from build123d import *

# Parameters (mm, degrees)
AUFSATZ_LINEAR_AUSTRAGEN1_DEPTH = 15
SKIZZE8_W                       = 15
SKIZZE8_H                       = 1.8
AUFSATZ_LINEAR_AUSTRAGEN2_DEPTH = 3.6
SKIZZE9_W                       = 1.8
SKIZZE9_H                       = 15
AUFSATZ_LINEAR_AUSTRAGEN3_DEPTH = 1.8
SKIZZE10_W                      = 1.8
SKIZZE10_H                      = 15
AUFSATZ_LINEAR_AUSTRAGEN4_DEPTH = 1.8


# Read off the part's stored shape, not the designer's step: Aufsatz-Linear austragen1
with BuildPart() as part:
    # Aufsatz-Linear austragen1 outline → Aufsatz-Linear austragen1 (new body)
    with BuildSketch(Plane.XY):
        with BuildLine():
            Line((9, 7.5), (9, 6.063801072))
            add(Edge.make_bspline(
                [(9, 6.063801072), (0.625422786, -0.579708044), (5, -9.5)],
                knots=[0.099237207, 0.099237207, 0.099237207, 1, 1, 1], degree=2))
            Line((5, -9.5), (5.897845721, -9.059689812))
            add(Edge.make_bspline(
                [(11, 6.296359693), (10.760549258, 6.131767377), (10.109849177, 5.669537639), (8.781306837, 4.626115655), (7.217816891, 3.118827009), (5.842447746, 1.269563984), (4.939494511, -0.621982734), (4.487436221, -2.56912246), (4.473192517, -4.602736578), (4.838873177, -6.401075315), (5.360722545, -7.892341674), (5.712043828, -8.68082614), (5.897845721, -9.059689812)],
                knots=[0.026920818, 0.026920818, 0.026920818, 0.026920818, 0.0625, 0.125, 0.25, 0.375, 0.5, 0.625, 0.75, 0.875, 0.9375, 1, 1, 1, 1], degree=3))
            Line((11, 6.296359693), (11, 9.5))
            Line((11, 9.5), (-1, 9.5))
            Line((-1, 9.5), (-1, -9.5))
            Line((-1, -9.5), (1, -9.5))
            Line((1, -9.5), (1, 7.5))
            Line((1, 7.5), (9, 7.5))
        make_face()
    extrude(amount=AUFSATZ_LINEAR_AUSTRAGEN1_DEPTH)

    # Skizze8 → Aufsatz-Linear austragen2 (add)
    with BuildSketch(Plane.ZY.offset(1)):
        with Locations((7.5, 8.6)):
            Rectangle(SKIZZE8_W, SKIZZE8_H)
        with Locations((7.5, -8.6)):
            Rectangle(SKIZZE8_W, SKIZZE8_H)
    extrude(amount=AUFSATZ_LINEAR_AUSTRAGEN2_DEPTH)

    # Skizze9 → Aufsatz-Linear austragen3 (add)
    with BuildSketch(Plane(origin=(0, -7.7, 0), x_dir=(1, 0, 0), z_dir=(0, 1, 0))):
        with Locations((-3.7, -7.5)):
            Rectangle(SKIZZE9_W, SKIZZE9_H)
    extrude(amount=AUFSATZ_LINEAR_AUSTRAGEN3_DEPTH)

    # Skizze10 → Aufsatz-Linear austragen4 (add)
    with BuildSketch(Plane.XZ.offset(-7.7)):
        with Locations((-3.7, 7.5)):
            Rectangle(SKIZZE10_W, SKIZZE10_H)
    extrude(amount=AUFSATZ_LINEAR_AUSTRAGEN4_DEPTH)


solid = part.part
Design review of the part built by this model. Coordinates are the model's own, in mm. A direction names the side the tool comes from. Give positions to 0.01 mm unless a question says otherwise; leave off trailing zeros. Order: outer loops, then holes, each group sorted by start corner. A loop starts at its lowest first (then second) coordinate and runs counter-clockwise, first axis right, second up. Notation, with made-up numbers: (26.5, 83.5) - (48.5, 83.5) arc R20 cw to (48.5, 94.5) - close; hole circle Ø2 at (84.5, 82). An arc over 180 degrees is marked (long way). Use CSV: the item, a comma, the result in double quotes. Start each with the question number.
Q1. For P1, Ø9, axis at x = 4.5, z = 4, coming from the -Y side; P2, Ø0.9, axis at y = -6.5, z = 8.5, coming from the +X side; P3, Ø7.5, axis at y = -0.5, z = 7.5, coming from the -X side, all flat-tipped, find the tip position at first contact; note any pin that passes through.
Q2. Take a section at D-D (x = 5.5). Count the separate pieces of the cut face and the enclosed holes in it, and give its area (3 significant figures).
Q3. Take a section at C-C (x = 1.25). State the section outline as (y, z) points.
Q4. Draft analysis for pull direction Y (two halves, no side actions). For faces 5 (the face through (-2.8, 7, 7)), 6 (the face through (0.85, 2.16, 15)), 7 (the face through (-4, -5.9, 7)), 8 (the face through (5.443, -9.283, 7.395)), state which applies: pulls with the +Y half, pulls with the -Y half, needs draft (parallel to the pull), parting line crosses it, or undercut.
Q5. Take a section at A-A (x = -3.5). State the section outline as (y, z) points.
Q6. Take a section at B-B (y = 7.25). State the section outline as (x, z) points, and give its area (3 significant figures).
Q7. For line 1 (Y direction, x = -1.5, z = 10.75); line 2 (X direction, y = -6, z = 1.75); line 3 (Y direction, x = -3.5, z = 12.5), list the stretches that pass through material, from the lowest coordinate up.
Q8. Machinability: for faces 1 (the face through (-4, 5.9, 8)), 2 (the face through (0.85, 2.16, 0)), 3 (the face through (1, -1, 7)), 4 (the face through (-1, 0, 7)), which of the approach directions +Z, -Z, +X, -X, +Y, -Y give a long, thin tool a straight path to every point of the face, cutting with its end or side? Answer none if there is none.
Calculated:
1,P1,"stops at y = -9.5"
1,P2,"stops at x = 5.04"
1,P3,"stops at x = -1"
2,separate pieces,"3"
2,enclosed holes,"0"
2,area,"75.1 mm²"
3,outline,"(7.5, 0) - (9.5, 0) - (9.5, 15) - (7.5, 15) - close"
4,face 5,"undercut"
4,face 6,"needs draft"
4,face 7,"undercut"
4,face 8,"pulls with the -Y half"
5,outline,"(-9.5, 0) - (-5.9, 0) - (-5.9, 15) - (-9.5, 15) - close; (5.9, 0) - (9.5, 0) - (9.5, 15) - (5.9, 15) - close"
6,outline,"(-4.6, 0) - (-2.8, 0) - (-2.8, 15) - (-4.6, 15) - close; (-1, 0) - (1, 0) - (1, 15) - (-1, 15) - close; (9, 0) - (11, 0) - (11, 15) - (9, 15) - close"
6,area,"87.0 mm²"
7,line 1,"y = -9.5 to -7.7, 7.7 to 9.5"
7,line 2,"x = -4.6 to -2.8, -1 to 1, 3.76 to 4.78"
7,line 3,"y = -9.5 to -5.9, 5.9 to 9.5"
8,face 1,"+Z, -Z, -X"
8,face 2,"-Z, +X, -X, +Y, -Y"
8,face 3,"+Z, -Z, -Y"
8,face 4,"+Z, -Z"
